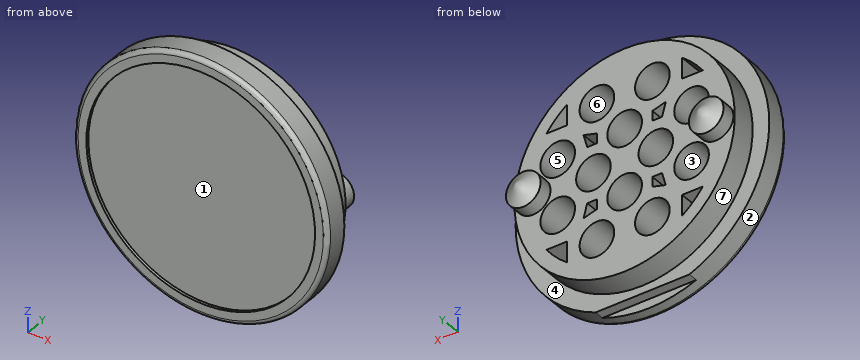
```python
from build123d import *

# Parameters (mm, degrees)
BOSS_EXTRUDE1_DEPTH      = 1.4
BOSS_EXTRUDE1_DEPTH_BACK = 0.3
SKETCH1_R                = 9.15
SKETCH2_R                = 8.25
CUT_EXTRUDE1_DEPTH       = 14
SKETCH3_R                = 7.95
BOSS_EXTRUDE2_DEPTH      = 1.8
SKETCH4_R                = 1.25
CUT_EXTRUDE2_DEPTH       = 14.405036367
SKETCH6_R                = 1.25
BOSS_EXTRUDE3_DEPTH      = 1
FILLET1_R                = 0.3
CUT_EXTRUDE6_START       = 0.7
SKETCH9_W                = 11.458380674
SKETCH9_H                = 2.677452805
CUT_EXTRUDE6_DEPTH       = 2
CROQUIS1_R               = 8.25
SALIENTE_EXTRUIR1_DEPTH  = 0.1


with BuildPart() as part:
    # Sketch1 → Boss-Extrude1 (new, two sides: drawn at the far end of the back side and taken through both)
    with BuildSketch(Plane(origin=(0, 0, 0), x_dir=(1, 0, 0), z_dir=(0, 1, 0)).offset(-BOSS_EXTRUDE1_DEPTH_BACK)):
        with Locations(Location((0, 0, 0), (0, 0, 270))):
            Circle(SKETCH1_R)
    extrude(amount=BOSS_EXTRUDE1_DEPTH + BOSS_EXTRUDE1_DEPTH_BACK)

    # Sketch2 → Cut-Extrude1 (cut)
    with BuildSketch(Plane(origin=(0, 0, 0), x_dir=(1, 0, 0), z_dir=(0, 1, 0))):
        with Locations(Location((0, 0, 0), (0, 0, 270))):
            Circle(SKETCH2_R)
    extrude(amount=-CUT_EXTRUDE1_DEPTH, mode=Mode.SUBTRACT)

    # Sketch3 → Boss-Extrude2 (add)
    with BuildSketch(Plane(origin=(0, 1.4, 0), x_dir=(1, 0, 0), z_dir=(0, 1, 0))):
        with Locations(Location((0, 0, 0), (0, 0, 270))):
            Circle(SKETCH3_R)
    extrude(amount=BOSS_EXTRUDE2_DEPTH)

    # Sketch4 → Cut-Extrude2 (cut, through all)
    with BuildSketch(Plane(origin=(0, 3.2, 0), x_dir=(1, 0, 0), z_dir=(0, 1, 0))):
        with Locations(Location((-2.25, 0, 0), (0, 0, 270))):
            Circle(SKETCH4_R)
        with Locations(Location((0, 2.25, 0), (0, 0, 270))):
            Circle(SKETCH4_R)
        with Locations(Location((-2, 4.828427125, 0), (0, 0, 270))):
            Circle(SKETCH4_R)
        with Locations(Location((-4.828427125, 2, 0), (0, 0, 270))):
            Circle(SKETCH4_R)
        with Locations(Location((4.828427125, 2, 0), (0, 0, 270))):
            Circle(SKETCH4_R)
        with Locations(Location((2, 4.828427125, 0), (0, 0, 270))):
            Circle(SKETCH4_R)
        with Locations(Location((2.25, 0, 0), (0, 0, 270))):
            Circle(SKETCH4_R)
        with Locations(Location((2, -4.828427125, 0), (0, 0, 270))):
            Circle(SKETCH4_R)
        with Locations(Location((4.828427125, -2, 0), (0, 0, 270))):
            Circle(SKETCH4_R)
        with Locations(Location((-4.828427125, -2, 0), (0, 0, 270))):
            Circle(SKETCH4_R)
        with Locations(Location((-2, -4.828427125, 0), (0, 0, 270))):
            Circle(SKETCH4_R)
        with Locations(Location((0, -2.25, 0), (0, 0, 270))):
            Circle(SKETCH4_R)
        with BuildLine():
            Line((-5.642596448, 4.142596448), (-4.142596448, 4.142596448))
            Line((-4.142596448, 4.142596448), (-4.142596448, 5.642596448))
            ThreePointArc((-4.142596448, 5.642596448), (-4.949747468, 4.949747468), (-5.642596448, 4.142596448))
        make_face()
        Polygon((-2.7, 2), (-2, 2), (-2, 2.7), (-2.964410286, 2.964410286), align=None)
        Polygon((2.964410286, 2.964410286), (2.7, 2), (2, 2), (2, 2.7), align=None)
        with BuildLine():
            Line((4.142596448, 5.642596448), (4.142596448, 4.142596448))
            Line((4.142596448, 4.142596448), (5.642596448, 4.142596448))
            ThreePointArc((5.642596448, 4.142596448), (4.949747468, 4.949747468), (4.142596448, 5.642596448))
        make_face()
        with BuildLine():
            Line((5.642596448, -4.142596448), (4.142596448, -4.142596448))
            Line((4.142596448, -4.142596448), (4.142596448, -5.642596448))
            ThreePointArc((4.142596448, -5.642596448), (4.949747468, -4.949747468), (5.642596448, -4.142596448))
        make_face()
        Polygon((2.7, -2), (2, -2), (2, -2.7), (2.964410286, -2.964410286), align=None)
        Polygon((-2.964410286, -2.964410286), (-2.7, -2), (-2, -2), (-2, -2.7), align=None)
        with BuildLine():
            Line((-4.142596448, -5.642596448), (-4.142596448, -4.142596448))
            Line((-4.142596448, -4.142596448), (-5.642596448, -4.142596448))
            ThreePointArc((-5.642596448, -4.142596448), (-4.949747468, -4.949747468), (-4.142596448, -5.642596448))
        make_face()
    extrude(amount=-CUT_EXTRUDE2_DEPTH, mode=Mode.SUBTRACT)

    # Sketch6 → Boss-Extrude3 (add)
    with BuildSketch(Plane(origin=(0, 3.2, 0), x_dir=(1, 0, 0), z_dir=(0, 1, 0))):
        with Locations(Location((-6.6, 0, 0), (0, 0, 270))):
            Circle(SKETCH6_R)
        with Locations(Location((6.6, 0, 0), (0, 0, 270))):
            Circle(SKETCH6_R)
    extrude(amount=BOSS_EXTRUDE3_DEPTH)

    # Sketch7 → Revolve1 (revolve)
    with BuildSketch(Plane.XY, mode=Mode.PRIVATE) as revolve1_sk:
        Polygon((-7.85, 4.2), (-6.6, 4.2), (-6.6, 4.9), align=None)
    revolve(revolve1_sk.sketch.rotate(Axis((-6.6, 4.2, 0), (0, 1, 0)), 270), axis=Axis((-6.6, 4.2, 0), (0, 1, 0)))

    # Sketch8 → Revolve2 (revolve)
    with BuildSketch(Plane.XY, mode=Mode.PRIVATE) as revolve2_sk:
        Polygon((7.85, 4.2), (6.6, 4.2), (6.6, 4.9), align=None)
    revolve(revolve2_sk.sketch.rotate(Axis((6.6, 4.2, 0), (0, 1, 0)), 90), axis=Axis((6.6, 4.2, 0), (0, 1, 0)))

    # Fillet1
    fillet1_edges = [part.edges().sort_by_distance(p)[0] for p in [
        (0, -0.3, -9.15),
    ]]
    fillet(fillet1_edges, radius=FILLET1_R - 0.0001)  # a hair under: the kernel refuses the full size

    # Sketch9 → Cut-Extrude6 (cut)
    with BuildSketch(Plane(origin=(0, 0, 0), x_dir=(1, 0, 0), z_dir=(0, 1, 0)).offset(CUT_EXTRUDE6_START)):
        with Locations((0, 9.838726403)):
            Rectangle(SKETCH9_W, SKETCH9_H)
    extrude(amount=CUT_EXTRUDE6_DEPTH, mode=Mode.SUBTRACT)

    # Croquis1 → Saliente-Extruir1 (add)
    with BuildSketch(Plane.XZ):
        with Locations(Location((0, 0, 0), (0, 0, 90))):
            Circle(CROQUIS1_R)
    extrude(amount=SALIENTE_EXTRUIR1_DEPTH)


solid = part.part
```
Here's how the part is built. I have some questions about the finished solid (model axes, mm). Face numbers are marked on the shaded views. A direction names the side the tool comes from. Coordinates: 2 decimals unless noted, no trailing zeros. Order: outer loops, then holes, each group sorted by start corner. A loop starts at its lowest first (then second) coordinate and runs counter-clockwise, first axis right, second up.
Item 1: I need wall thicknesses on probe 1 along X at (y, z) = (1.3, 2.5); probe 2 along X at (y, z) = (3.15, 4.5); probe 3 along X at (y, z) = (1.85, 2.25). Which ranges of each line are inside material? Lowest first, please.
Response values:
probe 1: x = -8.8 to -5.97, -3.68 to -2.84, -2 to -1.22, 1.22 to 2, 2.84 to 3.68, 5.97 to 8.8
probe 2: x = -6.55 to -5.36, -4.14 to -3.21, -0.79 to 0.79, 3.21 to 4.14, 5.36 to 6.55
probe 3: x = -7.62 to -6.05, -3.6 to -2.77, -2 to -1.25, 1.25 to 2, 2.77 to 3.6, 6.05 to 7.62
Item 2: If we section it at A-A, the plane x = 0: List the corners of the cut face in (y, z) for me, then the cut area to 3 significant figures.
Response values:
outline: (-0.3, -8.85) arc R0.3 ccw to (0, -9.15) - (0.7, -9.15) - (0.7, -8.5) - (1.4, -8.5) - (1.4, -7.95) - (3.2, -7.95) - (3.2, -3.5) - (0, -3.5) - (0, -1) - (3.2, -1) - (3.2, 1) - (0, 1) - (0, 3.5) - (3.2, 3.5) - (3.2, 7.95) - (1.4, 7.95) - (1.4, 9.15) - (0, 9.15) arc R0.3 ccw to (-0.3, 8.85) - (-0.3, 8.25) - (-0.1, 8.25) - (-0.1, -8.25) - (-0.3, -8.25) - close
area: 39.9 mm2
Item 3: I'm going to push flat-ended pins straight in: pin 1 Ø3 at (x, z) = (2.25, 0) entering from -Y; pin 2 Ø1.2 at (x, y) = (5, 1.5) entering from +Z; pin 3 Ø0.5 at (x, z) = (-2.5, 2.5) entering from +Y; pin 4 Ø1.5 at (y, z) = (4.5, -5) entering from -X. Where does each tip first touch, or does it pass through?
Response values:
pin 1: stops at y = -0.1
pin 2: stops at z = 8.02
pin 3: stops at y = 0
pin 4: passes through
Item 4: Which directions (+Z, -Z, +X, -X, +Y, -Y) give clear straight access to the entire face, cutting with the end or side of a thin tool? Please do the marked faces 1, 2 and 3.
Response values:
face 1: -Y
face 2: +Y, -Y
face 3: +Y
Item 5: Thinking about a two-plate mould opening in X: for the marked faces 4, 5, 6 and 7, which applies, pulls with the +X half, pulls with the -X half, needs draft (parallel to the pull), parting line crosses it, or undercut?
Response values:
face 4: needs draft
face 5: undercut
face 6: undercut
face 7: parting line crosses it
Item 6: If we section it at B-B, the plane y = 2.6: Give the number of separate pieces and of enclosed holes in the cut face, then the cut area to 3 significant figures.
Response values:
separate pieces: 1
enclosed holes: 20
area: 132 mm2
